Answer from the drawing. Dimensions are ordinates in mm from the lowest x, y and z of the part. A direction names the side the tool comes from. Round coordinates to 2 decimals unless told otherwise and drop trailing zeros. Loops run counter-clockwise (first coordinate to the right, second up) from the corner with the lowest first, then second, coordinate; pieces in that order, holes last.
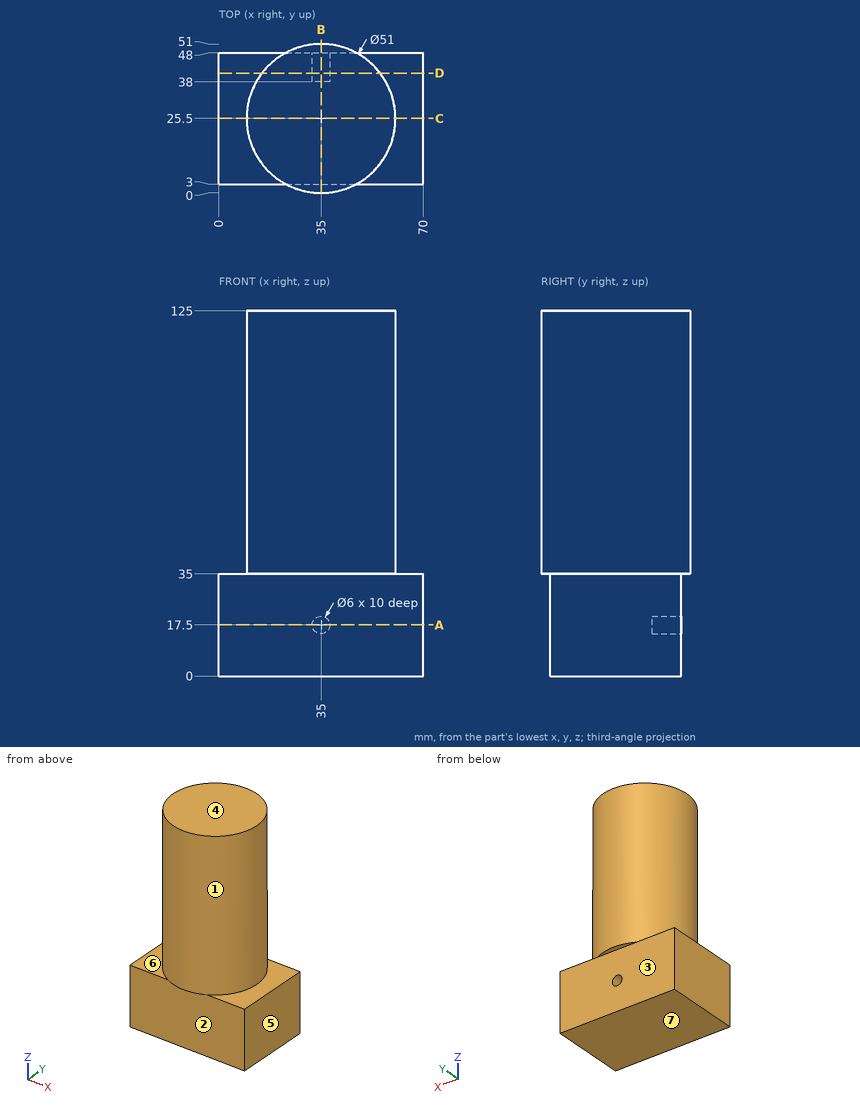
1. Which of the six approach directions +Z, -Z, +X, -X, +Y, -Y give full straight-line access (tool end or side, diameter ignored) to the marked faces 1, 2, 3 and 4?
Answer key:
face 1: +Z
face 2: -Z, +X, -X, -Y
face 3: -Z, +X, -X, +Y
face 4: +Z, +X, -X, +Y, -Y
2. Determine the mould class of the marked faces 5, 6 and 7 for opening direction Z: +Z half, -Z half, draft (parallel to the pull), parting line (faces both ways), or undercut.
Answer key:
face 5: draft
face 6: +Z half
face 7: -Z half
3. Find section D-D (y = 41). Write down the section's boundary in (x, z), then the cut area to 3 significant figures.
Answer key:
outline: (0, 0) - (70, 0) - (70, 35) - (55.25, 35) - (55.25, 125) - (14.75, 125) - (14.75, 35) - (0, 35) - close; hole circle Ø6 at (35, 17.5)
area: 6,070 mm2
4. Find section C-C (y = 25.5). Write down the section's boundary in (x, z).
Answer key:
outline: (0, 0) - (70, 0) - (70, 35) - (60.5, 35) - (60.5, 125) - (9.5, 125) - (9.5, 35) - (0, 35) - close
5. Find section B-B (x = 35). Write down the section's boundary in (y, z).
Answer key:
outline: (0, 35) - (3, 35) - (3, 0) - (48, 0) - (48, 14.5) - (38, 14.5) - (38, 20.5) - (48, 20.5) - (48, 35) - (51, 35) - (51, 125) - (0, 125) - close
6. Given pin 1 (2 mm diameter, centred on x = 26.5, z = 101.5, fed in from +Y); pin 2 (1.5 mm diameter, centred on x = 41, y = 2, fed in from -Z); pin 3 (10.5 mm diameter, centred on x = 23, z = 12, fed in from -Y), each flat-ended and moving along its own axis, determine where each tip first touches the part or whether it passes through.
Answer key:
pin 1: stops at y = 49.87
pin 2: stops at z = 35
pin 3: stops at y = 3
7. Consider probe 1 along Z at (x, y) = (35, 44); probe 2 along X at (y, z) = (40.5, 17.5); probe 3 along Z at (x, y) = (62, 23). Determine where each line is inside the solid, lowest interval first.
Answer key:
probe 1: z = 0 to 14.5, 20.5 to 125
probe 2: x = 0 to 32, 38 to 70
probe 3: z = 0 to 35
8. Find section A-A (z = 17.5). Write down the section's boundary in (x, y).
Answer key:
outline: (0, 3) - (70, 3) - (70, 48) - (38, 48) - (38, 38) - (32, 38) - (32, 48) - (0, 48) - close
